Can you work these out from the drawing? Everything is in mm from the part's minimum corner. A direction names the side the tool comes from. Round coordinates to 2 decimals unless told otherwise and drop trailing zeros. Write each loop counter-clockwise with the first axis right and the second up, starting at its lowest first coordinate (ties: lowest second). Pieces come first, ordered by that corner, then holes.
Q1. If we section it at D-D (y = 76.5): Please give me the cut outline in (x, z), plus the area to 3 significant figures.
Q2. Please list where these lines run through material, in increasing order: line 1 along Y through (x, z) = (152, 7); line 2 along X through (y, z) = (5, 16.5); line 3 along Z through (x, y) = (98, 28).
Q3. If we section it at A-A (x = 76.2): Please give me the cut outline in (y, z).
Q4. For the marked faces 4 and 5, which set-ups out of +Z, -Z, +X, -X, +Y, -Y let a thin tool reach every point of the face, with its end or its side?
Q5. I'm going to push a flat-ended pin straight in: pin 1 Ø2 at (x, y) = (78.5, 9) entering from +Z. Where does the tip first touch, or does it pass through?
Q6. If we section it at C-C (x = 109.5): Please give me the cut outline in (y, z).
Q7. We'd pull the mould along X, two halves only. Please class the marked faces 1, 2 and 3: +X half, -X half, draft (parallel to the pull), parting line (faces both ways), or undercut.
Q8. If we section it at B-B (z = 65.5): Please give me the cut outline in (x, y), plus the area to 3 significant figures.
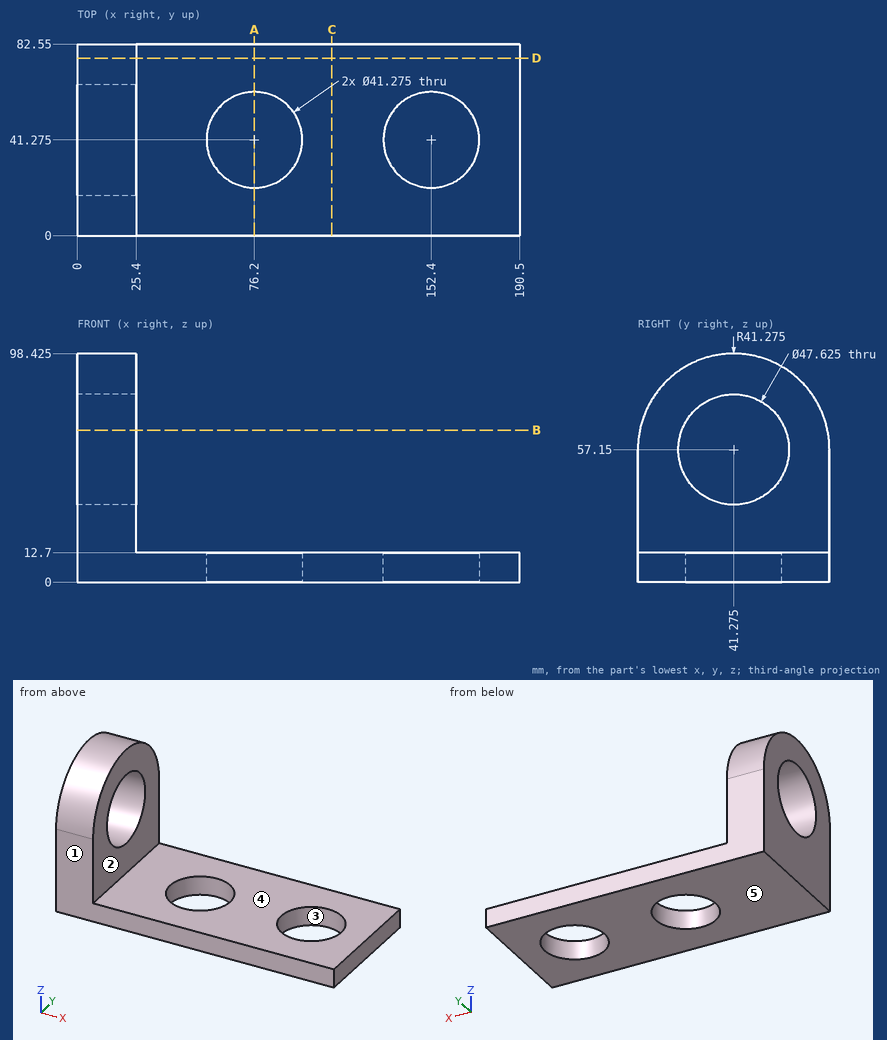
A:
1. outline: (0, 0) - (190.5, 0) - (190.5, 12.7) - (25.4, 12.7) - (25.4, 78.66) - (0, 78.66) - close
1. area: 4,090 mm2
2. line 1: y = 0 to 20.64, 61.91 to 82.55
2. line 2: x = 0 to 25.4
2. line 3: z = 0 to 12.7
3. outline: (0, 0) - (20.64, 0) - (20.64, 12.7) - (0, 12.7) - close; (61.91, 0) - (82.55, 0) - (82.55, 12.7) - (61.91, 12.7) - close
4. face 4: +Z, +X, +Y, -Y
4. face 5: -Z, +X, -X, +Y, -Y
5. pin 1: stops at z = 12.7
6. outline: (0, 0) - (82.55, 0) - (82.55, 12.7) - (0, 12.7) - close
7. face 1: draft
7. face 2: +X half
7. face 3: undercut
8. outline: (0, 0.85) - (25.4, 0.85) - (25.4, 18.97) - (0, 18.97) - close; (0, 63.58) - (25.4, 63.58) - (25.4, 81.7) - (0, 81.7) - close
8. area: 921 mm2
